Study the drawing (mm; zero at the part's minimum x, y, z) and answer. A direction names the side the tool comes from. Coordinates: 2 decimals unless noted, no trailing zeros. Order: outer loops, then holes, each group sorted by start corner. A loop starts at its lowest first (then second) coordinate and runs counter-clockwise, first axis right, second up. Notation, with made-up numbers: M 69,73 L 118,73 A31 ccw 118,110 Z; hole C 82,-9.5 d4. An arc over 180 degrees is marked long. Put each result on its own line as item: value.
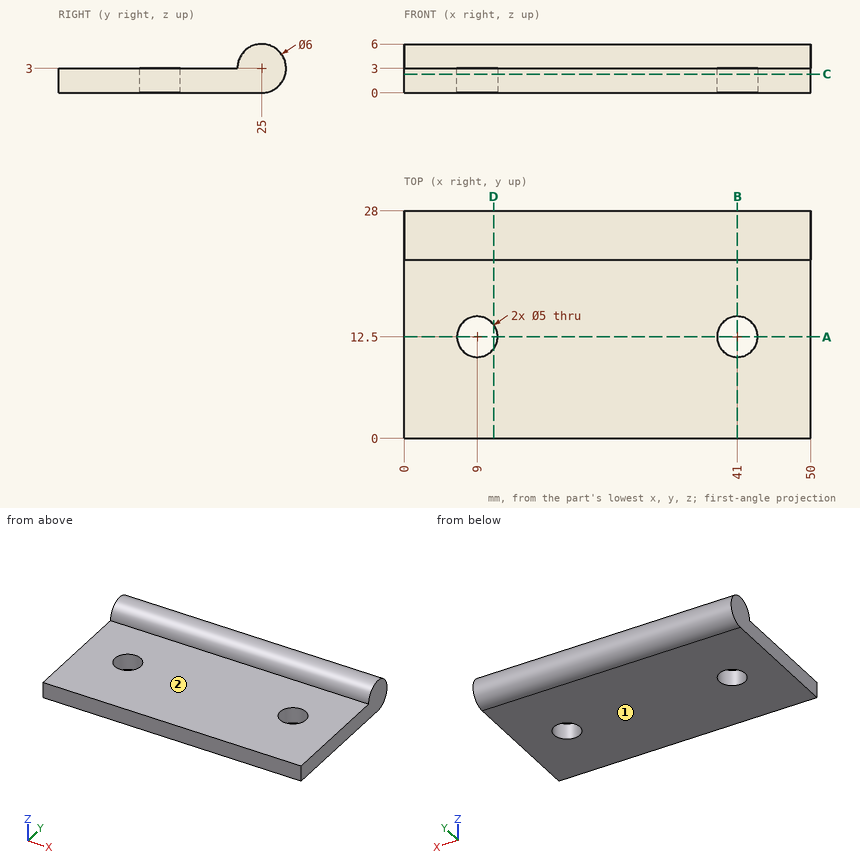
Q1. Find section C-C on z = 2.3. Write down the section's boundary in (x, y).
Answers below:
outline: M 0,0 L 50,0 L 50,27.92 L 0,27.92 Z; hole C 9,12.5 d5; hole C 41,12.5 d5
Q2. Find section D-D on x = 11. Write down the section's boundary in (y, z), plus the area to 3 significant figures.
Answers below:
outline: M 0,0 L 11,0 L 11,3 L 0,3 Z; M 14,0 L 25,0 A3 ccw long 22,3 L 14,3 Z
area: 87.2 mm^2
Q3. Find section A-A on y = 12.5. Write down the section's boundary in (x, z).
Answers below:
outline: M 0,0 L 6.5,0 L 6.5,3 L 0,3 Z; M 11.5,0 L 38.5,0 L 38.5,3 L 11.5,3 Z; M 43.5,0 L 50,0 L 50,3 L 43.5,3 Z
Q4. Given pin 1 (1 mm diameter, centred on x = 34, z = 5, fed in from +Y); pin 2 (2 mm diameter, centred on x = 44.5, z = 2, fed in from -Y); pin 3 (10 mm diameter, centred on x = 29.5, y = 11.5, fed in from +Z), each flat-ended and moving along its own axis, determine where each tip first touches the part or whether it passes through.
Answers below:
pin 1: stops at y = 27.6
pin 2: stops at y = 0
pin 3: stops at z = 3
Q5. Consider line 1 along Z through (x, y) = (16, 6.75); line 2 along Y through (x, z) = (29, 3.2); line 3 along Y through (x, z) = (9, 2.4). Determine where each line is inside the solid, lowest interval first.
Answers below:
line 1: z = 0 to 3
line 2: y = 22.01 to 27.99
line 3: y = 0 to 10, 15 to 27.94
Q6. A tool of negligible diameter and unlimited length cuts with its end or side. For the marked faces 1 and 2, from which of +Z, -Z, +X, -X, +Y, -Y can it reach the whole face along a straight path? Write none if from no direction.
Answers below:
face 1: -Z, +X, -X, +Y, -Y
face 2: +Z, +X, -X, -Y
Q7. Find section B-B on x = 41. Write down the section's boundary in (y, z), plus the area to 3 significant figures.
Answers below:
outline: M 0,0 L 10,0 L 10,3 L 0,3 Z; M 15,0 L 25,0 A3 ccw long 22,3 L 15,3 Z
area: 81.2 mm^2
